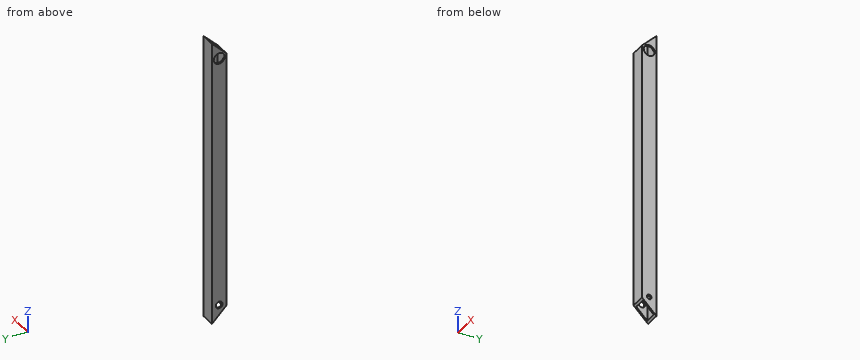
Autodesk Inventor part; units mm, degrees
ref_plane "YZ Plane" through (0, 0, 0) normal (1, 0, 0) x (0, 1, 0)
ref_plane "XZ Plane" through (0, 0, 0) normal (0, 1, 0) x (-1, 0, 0)
ref_plane "XY Plane" through (0, 0, 0) normal (0, 0, 1) x (1, 0, 0)
sketch "Sketch1" plane through (0, 0, 0) normal (0, 0, 1) x (1, 0, 0)
  line L0 (0, 0) -> (25, 0)
  line L1 (25, 0) -> (25, 25)
  line L2 (25, 25) -> (0, 25)
  line L3 (0, 25) -> (0, 0)
  line L4 (3, 22) -> (22, 22)
  line L5 (22, 22) -> (22, 3)
  line L6 (22, 3) -> (3, 3)
  line L7 (3, 3) -> (3, 22)
  dimension "d0" = 25
  dimension "d1" = 25
  dimension "d2" = 3
extrude "Extrusion1" add sketch "Sketch1" along normal blind 500
sketch "Sketch2" plane through (25, 0, 0) normal (1, 0, 0) x (0, 0, -1)
  line L0 (0, 0) -> (0, 25)
  line L1 (0, 25) -> (-500, 25)
  line L2 (-500, 0) -> (-500, 25)
  line L3 (0, 0) -> (-500, 0)
  line L4 (-500, 25) -> (-475, 0)
  line L5 (-500, 25) -> (-464.6447, 25) construction
  line L6 (0, 25) -> (-25, 0)
  line L7 (0, 25) -> (35.3553, 25) construction
  dimension "d5" = 45
  dimension "d6" = 135
extrude "Extrusion2" cut sketch "Sketch2" against normal blind 500 contours L3 L6 L0 | L4 L3 L2
sketch "Sketch3" plane through (25, 25, 500) normal (1, 0, 0) x (0, 0, -1)
  line L0 (475, -25) -> (25, -25)
  line L1 (500, 0) -> (0, 0)
  point P0 (500, -25)
  point P1 (30, -12.5)
  point P2 (470, -12.5)
  point P3 (250, 0)
  dimension "d9" = 440
  dimension "d10" = 12.5
  dimension "d11" = 220
hole "Hole1" at (25, 12.5, 30) direction (-1, 0, 0) diameter 8 depth 8 tip angle 118
sketch "Sketch5" plane through (0, 25, 0) normal (-1, 0, 0) x (0, 0, 1)
  circle A0 centre (30, -12.5) radius 4
  point P0 (0, -25)
  point P1 (470, -12.5)
  dimension "d33" = 440
hole "Hole3" at (0, 12.5, 30) at (0, 12.5, 470) direction (1, 0, 0) diameter 12 depth 8 tip angle 118
sketch "Sketch6" plane through (0, 25, 0) normal (-1, 0, 0) x (0, 0, 1)
  circle A0 centre (470, -12.5) radius 6
  point P0 (0, -25)
hole "Hole4" at (0, 12.5, 470) direction (1, 0, 0) diameter 19 end through all
properties part number "P501" material "Aluminum 6061"
Input: part model. Units: mm. Frame: model coordinates. Round coordinates to 2 decimals unless told otherwise and drop trailing zeros. Order: outer loops, then holes, each group sorted by start corner. A loop starts at its lowest first (then second) coordinate and runs counter-clockwise, first axis right, second up.
1. Cut plane A-A, the plane x = 17.25. Output: boundary loops of the cut face in (y, z), then the cut area to 3 significant figures.
The answers:
outline: (0, 25) - (3, 22) - (3, 478) - (0, 475) - close; (22, 3) - (25, 0) - (25, 500) - (22, 497) - close
area: 2,850 mm2
2. Cut plane B-B, the plane y = 12.5. Output: boundary loops of the cut face in (x, z), then the cut area to 3 significant figures.
The answers:
outline: (0, 12.5) - (3, 12.5) - (3, 24) - (0, 24) - close; (0, 36) - (3, 36) - (3, 460.5) - (0, 460.5) - close; (0, 479.5) - (3, 479.5) - (3, 487.5) - (0, 487.5) - close; (22, 12.5) - (25, 12.5) - (25, 26) - (22, 26) - close; (22, 34) - (25, 34) - (25, 460.5) - (22, 460.5) - close; (22, 479.5) - (25, 479.5) - (25, 487.5) - (22, 487.5) - close
area: 2,680 mm2
3. Material intervals for line 1 (Y direction, x = 1.5, z = 470); line 2 (Y direction, x = 23.1, z = 30); line 3 (Z direction, x = 1.5, y = 12.5), sorted ascending.
The answers:
line 1: y = 0 to 3, 22 to 25
line 2: y = 0 to 8.5, 16.5 to 25
line 3: z = 12.5 to 24, 36 to 460.5, 479.5 to 487.5
4. Pin query (flat end, axial travel): P1, Ø7, axis at y = 12.5, z = 30, coming from the +X side; P2, Ø1, axis at x = 19, z = 439, coming from the -Y side; P3, Ø6, axis at x = 3, y = 7.5, coming from the +Z side; P4, Ø10, axis at x = 21, y = 15, coming from the -Z side. Return the tip coordinate at first contact, or that it passes through.
The answers:
P1: passes through
P2: stops at y = 0
P3: stops at z = 485.5
P4: stops at z = 5.1
5. Cut plane C-C, the plane z = 376. Output: boundary loops of the cut face in (x, y), then the cut area to 3 significant figures.
The answers:
outline: (0, 0) - (25, 0) - (25, 25) - (0, 25) - close; hole (3, 3) - (22, 3) - (22, 22) - (3, 22) - close
area: 264 mm2
